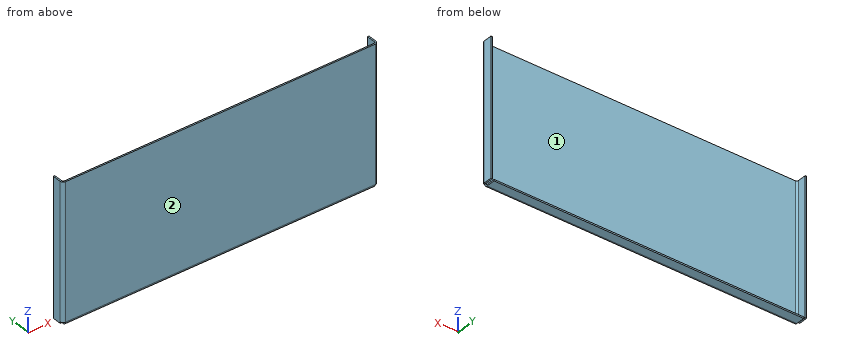
```python
from build123d import *

# Parameters (mm, degrees)
SKETCH1_W                      = 673.11016
SKETCH1_H                      = 290.83
BASE_FLANGE1_DEPTH             = 3.175
EDGE_FLANGE2_STRIP_W           = 19.05
EDGE_FLANGE2_STRIP_H           = 3.175
EDGE_FLANGE2_STRIP_CUT_DEPTH   = 290.83
EDGE_FLANGE2_STRIP_2_W         = 19.05
EDGE_FLANGE2_STRIP_2_H         = 3.175
EDGE_FLANGE2_STRIP_CUT_2_DEPTH = 290.83
EDGE_FLANGE2_DEPTH             = 290.83
EDGE_FLANGE2_BEND_DEPTH        = 290.83
EDGE_FLANGE3_DEPTH             = 673.11016
EDGE_FLANGE3_2_DEPTH           = 6.35
EDGE_FLANGE3_START             = 666.76016
EDGE_FLANGE3_3_DEPTH           = 6.35
EDGE_FLANGE3_START_2           = 6.35
EDGE_FLANGE3_4_DEPTH           = 660.41016


# Read off the part's stored shape, not the designer's step: Edge-Flange3
# Sheet-metal steps are written as plain solids
with BuildPart() as part:
    # Sketch1 → Base-Flange1 (new body)
    with BuildSketch(Plane(origin=(0, 0, 0), x_dir=(1, 0, 0), z_dir=(0, 1, 0))):
        with Locations((336.55508, 145.415)):
            Rectangle(SKETCH1_W, SKETCH1_H)
    extrude(amount=-BASE_FLANGE1_DEPTH)

    # Edge-Flange2 strip (across the edge) → Edge-Flange2 strip cut (cut)
    with BuildSketch(Plane(origin=(673.11016, 0, 0), x_dir=(-1, 0, 0), z_dir=(0, 0, -1))):
        with Locations((-3.175, -1.5875)):
            Rectangle(EDGE_FLANGE2_STRIP_W, EDGE_FLANGE2_STRIP_H)
    extrude(amount=EDGE_FLANGE2_STRIP_CUT_DEPTH, mode=Mode.SUBTRACT)

    # Edge-Flange2 strip 2 (across the edge) → Edge-Flange2 strip cut 2 (cut)
    with BuildSketch(Plane.XY.offset(-290.83)):
        with Locations((-3.175, -1.5875)):
            Rectangle(EDGE_FLANGE2_STRIP_2_W, EDGE_FLANGE2_STRIP_2_H)
    extrude(amount=EDGE_FLANGE2_STRIP_CUT_2_DEPTH, mode=Mode.SUBTRACT)

    # Edge-Flange2 section (across the edge) → Edge-Flange2 (add)
    with BuildSketch(Plane(origin=(673.11016, 0, 0), x_dir=(-1, 0, 0), z_dir=(0, 0, -1))):
        with BuildLine():
            Line((0, 3.175), (0, 22.225))
            Line((0, 22.225), (3.175, 22.225))
            Line((3.175, 22.225), (3.175, 3.175))
            ThreePointArc((3.175, 3.175), (4.10493597, 0.92993597), (6.35, 0))
            Line((6.35, 0), (6.35, -3.175))
            ThreePointArc((6.35, -3.175), (1.859871939, -1.315128061), (0, 3.175))
        make_face()
    extrude(amount=EDGE_FLANGE2_DEPTH)

    # Edge-Flange2 section 2 (across the edge) → Edge-Flange2 bend (add)
    with BuildSketch(Plane.XY.offset(-290.83)):
        with BuildLine():
            Line((0, 3.175), (0, 22.225))
            Line((0, 22.225), (3.175, 22.225))
            Line((3.175, 22.225), (3.175, 3.175))
            ThreePointArc((3.175, 3.175), (4.10493597, 0.92993597), (6.35, 0))
            Line((6.35, 0), (6.35, -3.175))
            ThreePointArc((6.35, -3.175), (1.859871939, -1.315128061), (0, 3.175))
        make_face()
    extrude(amount=EDGE_FLANGE2_BEND_DEPTH)

    # Edge-Flange3 outline → Edge-Flange3 (cut)
    with BuildSketch(Plane.YZ):
        with BuildLine():
            Line((3.175, -290.83), (3.175, -287.655))
            Line((3.175, -287.655), (0, -287.655))
            ThreePointArc((0, -287.655), (0.92993597, -289.90006403), (3.175, -290.83))
        make_face()
        with BuildLine():
            ThreePointArc((-2.324261315, -290.83), (-2.958628997, -289.298500936), (-3.175, -287.655))
            Line((-3.175, -287.655), (-3.175, -290.83))
            Line((-3.175, -290.83), (-2.324261315, -290.83))
        make_face()
    extrude(amount=EDGE_FLANGE3_DEPTH, mode=Mode.SUBTRACT)

    # Edge-Flange3 2 outline → Edge-Flange3 2 (cut)
    with BuildSketch(Plane.YZ):
        with BuildLine():
            ThreePointArc((3.175, -290.83), (0.92993597, -289.90006403), (0, -287.655))
            Line((0, -287.655), (-3.175, -287.655))
            ThreePointArc((-3.175, -287.655), (-2.958628997, -289.298500936), (-2.324261315, -290.83))
            Line((-2.324261315, -290.83), (3.175, -290.83))
        make_face()
    extrude(amount=EDGE_FLANGE3_2_DEPTH, mode=Mode.SUBTRACT)

    # Edge-Flange3 3 outline → Edge-Flange3 3 (cut)
    with BuildSketch(Plane.YZ.offset(EDGE_FLANGE3_START)):
        with BuildLine():
            ThreePointArc((3.175, -290.83), (0.92993597, -289.90006403), (0, -287.655))
            Line((0, -287.655), (-3.175, -287.655))
            ThreePointArc((-3.175, -287.655), (-2.958628997, -289.298500936), (-2.324261315, -290.83))
            Line((-2.324261315, -290.83), (3.175, -290.83))
        make_face()
    extrude(amount=EDGE_FLANGE3_3_DEPTH, mode=Mode.SUBTRACT)

    # Edge-Flange3 4 outline → Edge-Flange3 4 (add)
    with BuildSketch(Plane.YZ.offset(EDGE_FLANGE3_START_2)):
        with BuildLine():
            Line((0, -287.655), (0, -290.83))
            Line((0, -290.83), (-2.324261315, -290.83))
            ThreePointArc((-2.324261315, -290.83), (-1e-09, -293.154261314), (3.175, -294.005))
            Line((3.175, -294.005), (22.225, -294.005))
            Line((22.225, -294.005), (22.225, -290.83))
            Line((22.225, -290.83), (3.175, -290.83))
            ThreePointArc((3.175, -290.83), (0.92993597, -289.90006403), (0, -287.655))
        make_face()
    extrude(amount=EDGE_FLANGE3_4_DEPTH)


solid = part.part
```
Design review of the part built by this model. Coordinates are the model's own, in mm. Face numbers are marked on the shaded views. Coordinates: 2 decimals unless noted, no trailing zeros. Loops run counter-clockwise (first coordinate to the right, second up) from the corner with the lowest first, then second, coordinate; pieces in that order, holes last.
Q1. We need section C-C on x = 436. State the section outline as (y, z) points (3 decimals), and give its area (3 significant figures).
Reported:
outline: (-3.175, -287.655) arc R6.35 ccw to (3.175, -294.005) - (22.225, -294.005) - (22.225, -290.83) - (3.175, -290.83) arc R3.175 cw to (0, -287.655) - (0, 0) - (-3.175, 0) - close
area: 998 mm2
Q2. The part is to be moulded in two halves that separate along X. For the marked faces 1 and 2, say which applies: +X half, -X half, draft (parallel to the pull), parting line (faces both ways), or undercut.
Reported:
face 1: undercut
face 2: draft
Q3. We need section B-B on z = -270. State the section outline as (x, y) points (3 decimals).
Reported:
outline: (0, 3.175) arc R6.35 ccw to (6.35, -3.175) - (666.76, -3.175) arc R6.35 ccw to (673.11, 3.175) - (673.11, 22.225) - (669.935, 22.225) - (669.935, 3.175) arc R3.175 cw to (666.76, 0) - (6.35, 0) arc R3.175 cw to (3.175, 3.175) - (3.175, 22.225) - (0, 22.225) - close
Q4. We need section A-A on y = 11.75. State the section outline as (x, z) points (3 decimals), and give its area (3 significant figures).
Reported:
outline: (0, -290.83) - (3.175, -290.83) - (3.175, 0) - (0, 0) - close; (6.35, -294.005) - (666.76, -294.005) - (666.76, -290.83) - (6.35, -290.83) - close; (669.935, -290.83) - (673.11, -290.83) - (673.11, 0) - (669.935, 0) - close
area: 3,940 mm2
Q5. For pin 1 (1.6 mm diameter, centred on x = 671, z = -290, fed in from -Y) (3 decimals); pin 2 (1 mm diameter, centred on x = 1, y = 17, fed in from -Z); pin 3 (3 mm diameter, centred on x = 670, y = 1, fed in from -Z) (3 decimals), all flat-tipped, find the tip position at first contact; note any pin that passes through.
Reported:
pin 1: stops at y = 3.175
pin 2: stops at z = -290.83
pin 3: stops at z = -287.655
Q6. To check wall thickness, follow line 1 (X direction, y = 8.75, z = -176.5) (3 decimals); line 2 (Y direction, x = 338.5, z = -231) (3 decimals); line 3 (X direction, y = 1.5, z = -187). State the ranges of each line that lie inside material, in increasing order.
Reported:
line 1: x = 0 to 3.175, 669.935 to 673.11
line 2: y = -3.175 to 0
line 3: x = 0.22 to 3.65, 669.46 to 672.89
